The drawing under review shows one solid part. Ordinate dimensions are in mm from its lowest x, y, z. A direction names the side the tool comes from. Coordinates: 2 decimals unless noted, no trailing zeros. Write each loop counter-clockwise with the first axis right and the second up, starting at its lowest first coordinate (ties: lowest second). Pieces come first, ordered by that corner, then holes. Notation, with made-up numbers: (67.25, 48.5) -> (102.25, 48.5) arc R29 cw to (102.25, 69.5) -> close; hole circle Ø4 at (-9.5, 41). An arc over 180 degrees is marked (long way). Put each result on its own line as item: value. Start each with the question number.
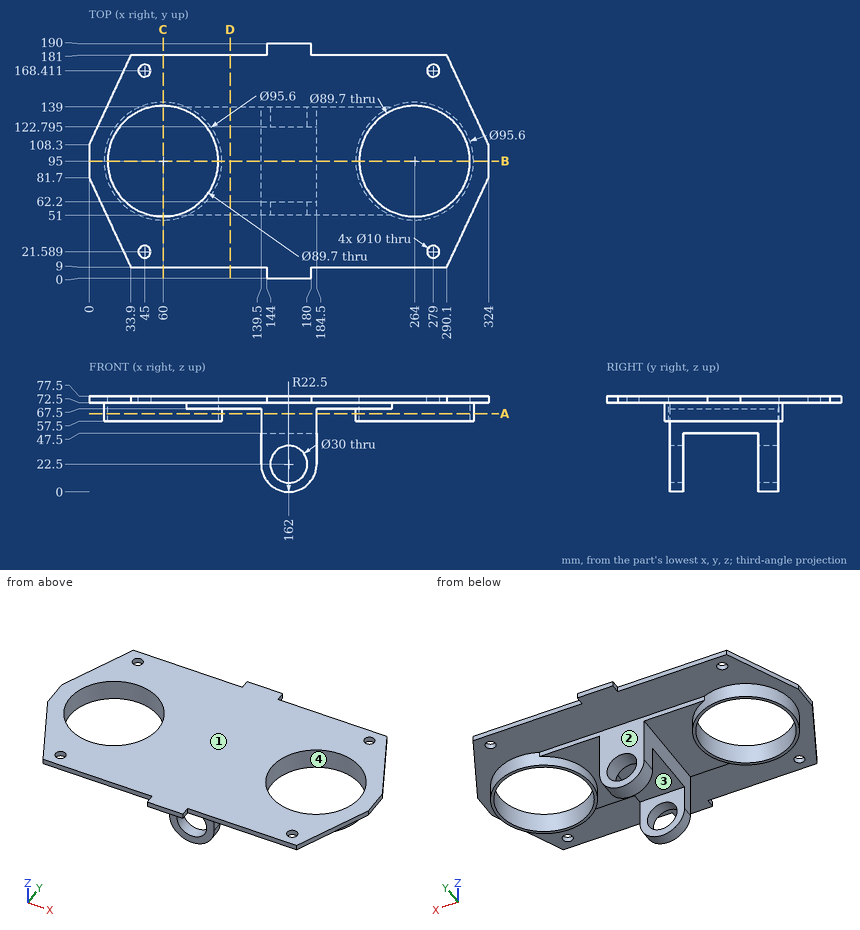
1. Consider section A-A on z = 63.5. State the section outline as (x, y) points.
2. Wall thickness on line 1 (X direction, y = 171, z = 73); line 2 (Y direction, x = 45, z = 75.3); line 3 (Z direction, x = 222, y = 48.5): over which ranges is each line inside the solid? List them lowest first. Write a range as from..to.
3. Consider section C-C on x = 60. State the section outline as (y, z) points, then the cut area to 3 significant figures.
4. Consider section D-D on x = 114.5. State the section outline as (y, z) points, then the cut area to 3 significant figures.
5. The part is to be moulded in two halves that separate along X. For the marked faces 1 and 2, say which applies: released by +X, released by -X, zero draft, split by the parting line, or undercut.
6. Tool access review of the marked faces 3 and 4: name each direction out of +Z, -Z, +X, -X, +Y, -Y from which nothing blocks a thin tool from reaching the whole face with its end or side.
7. Insertion check: P1, Ø10, axis at y = 116, z = 69.5, coming from the -X side (1 decimal); P2, Ø1.5, axis at x = 180.5, z = 22.5, coming from the +Y side; P3, Ø2.5, axis at y = 185, z = 74, coming from the +X side. Each pin has a flat end and moves straight along its axis. Give the tip position at first contact, or say it passes through.
8. Consider section B-B on y = 95. State the section outline as (x, z) points, then the cut area to 3 significant figures.
Output values:
1. outline: circle Ø95.6 at (60, 95); (139.5, 51) -> (184.5, 51) -> (184.5, 139) -> (139.5, 139) -> close; circle Ø95.6 at (264, 95); hole circle Ø89.7 at (60, 95); hole circle Ø89.7 at (264, 95)
2. line 1: x = 29.24..40.72, 49.28..274.72, 283.28..294.76
2. line 2: y = 9..16.59, 26.59..52.73, 137.27..163.41, 173.41..181
2. line 3: z = 72.5..77.5
3. outline: (9, 72.5) -> (47.2, 72.5) -> (47.2, 57.5) -> (50.15, 57.5) -> (50.15, 77.5) -> (9, 77.5) -> close; (139.85, 57.5) -> (142.8, 57.5) -> (142.8, 72.5) -> (181, 72.5) -> (181, 77.5) -> (139.85, 77.5) -> close
3. area: 500 mm^2
4. outline: (9, 72.5) -> (51, 72.5) -> (51, 67.5) -> (139, 67.5) -> (139, 72.5) -> (181, 72.5) -> (181, 77.5) -> (9, 77.5) -> close
4. area: 1,300 mm^2
5. face 1: zero draft
5. face 2: undercut
6. face 3: -Z, +X, -X
6. face 4: +Z, -Z
7. P1: stops at x = 1.7
7. P2: stops at y = 139
7. P3: stops at x = 180
8. outline: (0, 72.5) -> (12.2, 72.5) -> (12.2, 57.5) -> (15.15, 57.5) -> (15.15, 77.5) -> (0, 77.5) -> close; (104.85, 57.5) -> (107.8, 57.5) -> (107.8, 67.5) -> (139.5, 67.5) -> (139.5, 47.5) -> (184.5, 47.5) -> (184.5, 67.5) -> (216.2, 67.5) -> (216.2, 57.5) -> (219.15, 57.5) -> (219.15, 77.5) -> (104.85, 77.5) -> close; (308.85, 57.5) -> (311.8, 57.5) -> (311.8, 72.5) -> (324, 72.5) -> (324, 77.5) -> (308.85, 77.5) -> close
8. area: 2,340 mm^2
